Autodesk Inventor part; units mm, degrees
ref_plane "YZ Plane" through (0, 0, 0) normal (1, 0, 0) x (0, 1, 0)
ref_plane "XZ Plane" through (0, 0, 0) normal (0, 1, 0) x (-1, 0, 0)
ref_plane "XY Plane" through (0, 0, 0) normal (0, 0, 1) x (1, 0, 0)
sketch "Sketch1" plane through (0, 0, 0) normal (0, 1, 0) x (-1, 0, 0)
  circle A0 centre (0, 0) radius 9.525
  dimension "d0" = 19.05
extrude "Extrusion1" add sketch "Sketch1" along normal blind 1.27
sketch "Sketch2" plane through (0, 1.27, 0) normal (0, 1, 0) x (1, 0, 0)
  line L0 (6.35, -3.6662) -> (0, -7.3323)
  line L1 (0, -7.3323) -> (-6.35, -3.6662)
  line L2 (-6.35, -3.6662) -> (-6.35, 3.6662)
  line L3 (-6.35, 3.6662) -> (0, 7.3323)
  line L4 (0, 7.3323) -> (6.35, 3.6662)
  line L5 (6.35, 3.6662) -> (6.35, -3.6662)
  point P0 (0, 0)
  point P1 (0, 0)
  dimension "d4" = 12.7
extrude "Extrusion2" add sketch "Sketch2" along normal blind 4.7625
fillet "Fillet1" radius 0.508 6 edges at (6.35, 3.6513, 3.6662) (6.35, 3.6513, -3.6662) (0, 3.6513, -7.3323) (0, 3.6513, 7.3323) (-6.35, 3.6513, 3.6662) (-6.35, 3.6513, -3.6662)
sketch "Sketch3" plane through (0, 6.0325, 0) normal (0, 1, 0) x (1, 0, 0)
  line L0 (-2.7178, -3.2258) -> (2.7178, -3.2258)
  line L1 (3.2258, -2.7178) -> (3.2258, 2.7178)
  line L2 (2.7178, 3.2258) -> (-2.7178, 3.2258)
  line L3 (-3.2258, 2.7178) -> (-3.2258, -2.7178)
  line L4 (-3.2258, -3.2258) -> (3.2258, 3.2258) construction
  line L5 (3.2258, -3.2258) -> (-3.2258, 3.2258) construction
  arc A0 (-3.2258, -2.7178) -> (-2.7178, -3.2258) centre (-2.7178, -2.7178) ccw
  arc A1 (2.7178, -3.2258) -> (3.2258, -2.7178) centre (2.7178, -2.7178) ccw
  arc A2 (3.2258, 2.7178) -> (2.7178, 3.2258) centre (2.7178, 2.7178) ccw
  arc A3 (-2.7178, 3.2258) -> (-3.2258, 2.7178) centre (-2.7178, 2.7178) ccw
  point P0 (0, 0)
  dimension "d8" = 6.4516
  dimension "d9" = 0.508
extrude "Extrusion3" cut sketch "Sketch3" against normal through all
chamfer "Chamfer1" distance 0.3969 angle 45 12 edges at (3.175, 1.27, -5.4993) (6.2819, 1.27, -3.6269) (6.35, 1.27, 0) (6.2819, 1.27, 3.6269) (3.175, 1.27, 5.4993) (0, 1.27, 7.2538) (-3.175, 1.27, 5.4993) (-6.2819, 1.27, 3.6269) (-6.35, 1.27, 0) (-6.2819, 1.27, -3.6269) (-3.175, 1.27, -5.4993) (0, 1.27, -7.2538)
properties part number "insert" material "Acetal Resin, Black"
Work out the finished part from the listing and answer in its coordinate system (mm). A direction names the side the tool comes from. Give positions to 0.01 mm unless a question says otherwise; leave off trailing zeros. Write each loop counter-clockwise with the first axis right and the second up, starting at its lowest first coordinate (ties: lowest second). Pieces come first, ordered by that corner, then holes.
(1) The part is cut by section D-D on x = 5. Write down the section's boundary in (y, z), plus the area to 3 significant figures.
Final values:
outline: (0, -8.11) - (1.27, -8.11) - (1.27, -4.9) - (1.67, -4.45) - (6.03, -4.45) - (6.03, 4.45) - (1.67, 4.45) - (1.27, 4.9) - (1.27, 8.11) - (0, 8.11) - close
area: 63.1 mm2
(2) Flat-ended cylindrical pins translate along their axes: pin 1 Ø2.5 at (x, y) = (0.5, 3) entering from +Z; pin 2 Ø2 at (y, z) = (3, 1.5) entering from -X; pin 3 Ø1.5 at (y, z) = (0.5, 4) entering from +X. Find the tip coordinate at first contact, or state that the pin passes through.
Final values:
pin 1: stops at z = 7.25
pin 2: stops at x = -6.35
pin 3: stops at x = 8.95
(3) The part is cut by section B-B on x = 0. Write down the section's boundary in (y, z) (1 decimal), plus the area to 3 significant figures.
Final values:
outline: (0, -9.5) - (1.3, -9.5) - (1.3, -7.7) - (1.7, -7.3) - (6, -7.3) - (6, -3.2) - (0, -3.2) - close; (0, 3.2) - (6, 3.2) - (6, 7.3) - (1.7, 7.3) - (1.3, 7.7) - (1.3, 9.5) - (0, 9.5) - close
area: 54.5 mm2
(4) The mould has two halves that part along Z. Classify faces 1 (the flat face through (3.31, 1.47, 5.65)), 2 (the flat face through (6.35, 4, 0)), 3 (the flat face through (-3.226, 3, 0)): pulls with the +Z half, pulls with the -Z half, needs draft (parallel to the pull), parting line crosses it, or undercut.
Final values:
face 1: pulls with the +Z half
face 2: needs draft
face 3: undercut
(5) Which of the six approach directions +Z, -Z, +X, -X, +Y, -Y give full straight-line access (tool end or side, diameter ignored) to faces 4 (the flat face through (-6.35, 4, 0)), 5 (the flat face through (-3.134, 3.819, 5.523)), 6 (the flat face through (0, 3, -3.226)), 7 (the flat face through (3.216, 3.819, 5.476))?
Final values:
face 4: +Z, -Z, -X, +Y
face 5: +Z, -X, +Y
face 6: +Y, -Y
face 7: +Z, +X, +Y
(6) The part is cut by section C-C on y = 5.75. Write down the section's boundary in (x, z).
Final values:
outline: (-6.35, -3.37) arc R0.51 ccw to (-6.1, -3.81) - (-0.25, -7.19) arc R0.51 ccw to (0.25, -7.19) - (6.1, -3.81) arc R0.51 ccw to (6.35, -3.37) - (6.35, 3.37) arc R0.51 ccw to (6.1, 3.81) - (0.25, 7.19) arc R0.51 ccw to (-0.25, 7.19) - (-6.1, 3.81) arc R0.51 ccw to (-6.35, 3.37) - close; hole (-3.23, -2.72) arc R0.51 ccw to (-2.72, -3.23) - (2.72, -3.23) arc R0.51 ccw to (3.23, -2.72) - (3.23, 2.72) arc R0.51 ccw to (2.72, 3.23) - (-2.72, 3.23) arc R0.51 ccw to (-3.23, 2.72) - close
(7) Straight lines are drawn through the part: line 1 (X direction, y = 5, z = 1.75); line 2 (Y direction, x = 8, z = -2.5); line 3 (Z direction, x = -2, y = 1). For each, find the intervals that lie inside material, in ascending order.
Final values:
line 1: x = -6.35 to -3.23, 3.23 to 6.35
line 2: y = 0 to 1.27
line 3: z = -9.31 to -3.23, 3.23 to 9.31
